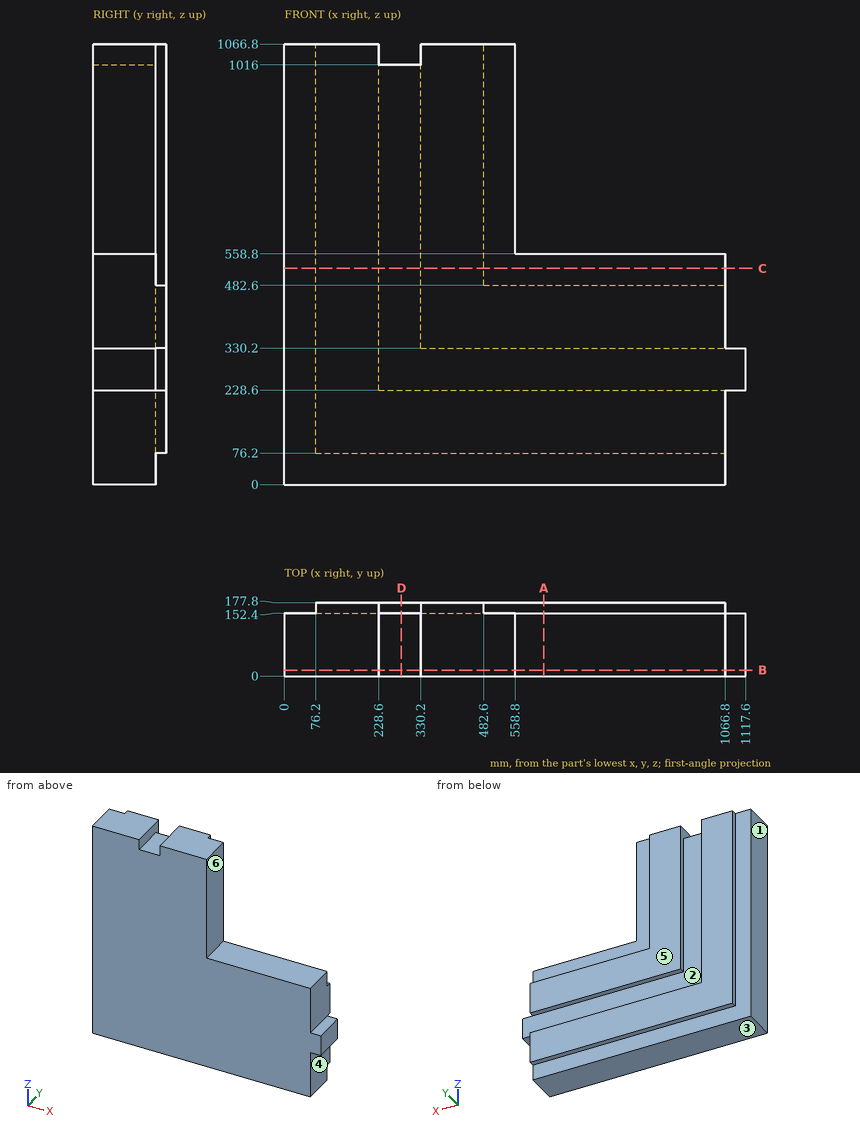
Can you work these out from the drawing? Everything is in mm from the part's minimum corner. A direction names the side the tool comes from. Give positions to 0.01 mm unless a question says otherwise; leave off trailing zeros. Write each loop counter-clockwise with the first axis right and the second up, starting at its lowest first coordinate (ties: lowest second). Pieces come first, ordered by that corner, then holes. Notation, with made-up numbers: (-31.5, 9.5) -> (-10.5, 9.5) arc R29 ccw to (-10.5, 31.5) -> close; hole circle Ø4 at (8, 31). An arc over 180 degrees is marked (long way). Write each question's results on one line, items separated by ' | '. Start each with the question number.
Q1. We'd pull the mould along X, two halves only. Please class the marked faces 1, 2 and 3: +X half, -X half, draft (parallel to the pull), parting line (faces both ways), or undercut.
Q2. Suppose I cut it at C-C, the plane z = 523.5. List the corners of the cut face in (x, y) for me.
Q3. I need wall thicknesses on probe 1 along Z at (x, y) = (1021, 153); probe 2 along X at (y, z) = (149.5, 945). Which ranges of each line are inside material? Lowest first, please.
Q4. Suppose I cut it at D-D, the plane x = 283. List the corners of the cut face in (y, z) for me.
Q5. I'm going to push flat-ended pins straight in: pin 1 Ø12.5 at (x, y) = (826, 160.5) entering from +Z; pin 2 Ø6 at (x, z) = (750.5, 522) entering from +Y; pin 3 Ø1 at (y, z) = (49, 494) entering from -X; pin 4 Ø20.5 at (x, y) = (658.5, 163.5) entering from -Z. Where does each tip first touch, or does it pass through?
Q6. Suppose I cut it at B-B, the plane y = 14. List the corners of the cut face in (x, z) for me.
Q7. Suppose I cut it at A-A, the plane x = 628. List the corners of the cut face in (y, z) for me, and give its area (3 significant figures).
Q8. Which directions (+Z, -Z, +X, -X, +Y, -Y) give clear straight access to the entire face, cutting with the end or side of a thin tool? Please do the marked faces 4, 5 and 6.
Outcome:
1) face 1: -X half | face 2: undercut | face 3: draft
2) outline: (0, 0) -> (1066.8, 0) -> (1066.8, 152.4) -> (482.6, 152.4) -> (482.6, 177.8) -> (330.2, 177.8) -> (330.2, 152.4) -> (228.6, 152.4) -> (228.6, 177.8) -> (76.2, 177.8) -> (76.2, 152.4) -> (0, 152.4) -> close
3) probe 1: 76.2 to 228.6, 330.2 to 482.6 | probe 2: 0 to 558.8
4) outline: (0, 0) -> (152.4, 0) -> (152.4, 76.2) -> (177.8, 76.2) -> (177.8, 228.6) -> (152.4, 228.6) -> (152.4, 1016) -> (0, 1016) -> close
5) pin 1: z = 482.6 | pin 2: y = 152.4 | pin 3: x = 0 | pin 4: z = 76.2
6) outline: (0, 0) -> (1066.8, 0) -> (1066.8, 228.6) -> (1117.6, 228.6) -> (1117.6, 330.2) -> (1066.8, 330.2) -> (1066.8, 558.8) -> (558.8, 558.8) -> (558.8, 1066.8) -> (330.2, 1066.8) -> (330.2, 1016) -> (228.6, 1016) -> (228.6, 1066.8) -> (0, 1066.8) -> close
7) outline: (0, 0) -> (152.4, 0) -> (152.4, 76.2) -> (177.8, 76.2) -> (177.8, 228.6) -> (152.4, 228.6) -> (152.4, 330.2) -> (177.8, 330.2) -> (177.8, 482.6) -> (152.4, 482.6) -> (152.4, 558.8) -> (0, 558.8) -> close | area: 92,900 mm2
8) face 4: -Z, +X, +Y, -Y | face 5: +Z, -Z, +X, -X, +Y | face 6: +Z, +X, +Y, -Y
